Check sheet for the modelled part. Datum: model origin and axes. Units: mm. A direction names the side the tool comes from. Coordinates: 2 decimals unless noted, no trailing zeros. Write each loop counter-clockwise with the first axis right and the second up, starting at its lowest first coordinate (ties: lowest second). Pieces come first, ordered by that corner, then holes. Notation, with made-up numbers: (42, -30) - (79, -30) arc R5 ccw to (79, -23) - close; hole circle Ø3 at (15.25, 64). An arc over 180 degrees is marked (long way). Use one line per item in the form item = value. Start each with the question number.
1. Cross-section at A-A on y = -21. Record the boundary of the cut face in (x, z), then the cut area to 3 significant figures.
2. Go/stop test with flat-tipped pins: pin 1 Ø1 at (x, z) = (-9, 3.5) entering from +Y; pin 2 Ø5 at (x, y) = (7.5, -29) entering from -Z; pin 3 Ø2 at (x, z) = (14, 11) entering from +Y. Record where each tip stops, or that it passes through.
3. Cross-section at C-C on z = -7.5. Record the boundary of the cut face in (x, y).
4. Tool access check on faces 1 (the face through (17, -29, 5.625)), 2 (the face through (-4.5, -29, -18)), 3 (the face through (18.47, -27.986, 7.625)), 4 (the face through (5.36, -30.27, -1.29)). Record the directions out of +Z, -Z, +X, -X, +Y, -Y that give a thin tool (end or side, any length) a straight path to the whole face; none if there is none.
5. Cross-section at B-B on y = -11. Record the boundary of the cut face in (x, z).
6. Draft check along Z on faces 5 (the face through (6.31, -27.99, 5.84)), 6 (the face through (-8, -18.95, 2)), 7 (the face through (17, -29, 14.625)). Enter one of: +Z half, -Z half, draft (parallel to the pull), parting line (faces both ways), or undercut.
7. Scan lines: line 1 along Z through (x, y) = (7.5, -29.6); line 2 along X through (y, z) = (-30.95, -17.75); line 3 along Y through (x, z) = (11.5, -4.5). Record each from-to range of solid material in increasing order.
```python
from build123d import *

# Parameters (mm, degrees)
F0_R          = 1.5
F0_R_2        = 4.25
F1_DEPTH      = 3.5
F2_R          = 1.5
F2_W          = 9
F2_H          = 9
F2_R_2        = 1.6
F2_W_2        = 25
F2_H_2        = 3.5
F3_DEPTH      = 3.5
F3_DEPTH_BACK = 1
F4_R          = 1.6
F5_DEPTH      = 2
F6_R          = 2.9
F6_R_2        = 1.5
F7_DEPTH      = 2.5


# Not quite as in the source:
# - a feature names something its author has since deleted; it is built from what else it names


with BuildPart() as f1:
    # F0 (on Top) → F1 (new body)
    with BuildSketch(Plane.XY):
        with BuildLine():
            Line((-14.1, -30.5), (0, -30.5))
            Line((0, -30.5), (14.1, -30.5))
            Line((14.1, -30.5), (14.1, -12))
            Line((14.1, -12), (9.025382269, 3.044355416))
            ThreePointArc((9.025382269, 3.044355416), (0, 9.525), (-9.025382269, 3.044355416))
            Line((-9.025382269, 3.044355416), (-14.1, -12))
            Line((-14.1, -12), (-14.1, -30.5))
        make_face()
        Polygon((10.2, -27), (0, -27), (-10.2, -27), (-10.2, -18.95), (-5, -18.95), (-5, -9.525), (0, -9.525), (5, -9.525), (5, -18.95), (10.2, -18.95), align=None, mode=Mode.SUBTRACT)
        with Locations((-5.499261314, 3.175)):
            Circle(F0_R, mode=Mode.SUBTRACT)
        with Locations((0, -6.35)):
            Circle(F0_R, mode=Mode.SUBTRACT)
        Circle(F0_R_2, mode=Mode.SUBTRACT)
        with Locations((5.499261314, 3.175)):
            Circle(F0_R, mode=Mode.SUBTRACT)
    extrude(amount=F1_DEPTH)

    # F2 (on face) → F3 (join, two sides)
    with BuildSketch(Plane.XZ.offset(30.5)) as f3_sk:
        Polygon((12.5, 16.75), (-12.5, 16.75), (-12.5, 14.625), (-12.5, 5.625), (-12.5, 3.5), (12.5, 3.5), (12.5, 5.625), (12.5, 14.625), align=None)
        with Locations((-7.5, 6.75)):
            Circle(F2_R, mode=Mode.SUBTRACT)
        with Locations((7.5, 6.75)):
            Circle(F2_R, mode=Mode.SUBTRACT)
        Polygon((12.5, 0), (-12.5, 0), (-12.5, -13.25), (-4.5, -13.25), (4.5, -13.25), (12.5, -13.25), align=None)
        with Locations((-7.5, -3.25)):
            Circle(F2_R, mode=Mode.SUBTRACT)
        with Locations((7.5, -3.25)):
            Circle(F2_R, mode=Mode.SUBTRACT)
        with Locations((-17, 10.125)):
            Rectangle(F2_W, F2_H)
        with Locations((-17, 10.125)):
            Circle(F2_R_2, mode=Mode.SUBTRACT)
        with Locations((17, 10.125)):
            Rectangle(F2_W, F2_H)
        with Locations((17, 10.125)):
            Circle(F2_R_2, mode=Mode.SUBTRACT)
        with Locations((0, -17.75)):
            Rectangle(F2_W, F2_H)
        with Locations((0, -17.75)):
            Circle(F2_R_2, mode=Mode.SUBTRACT)
        with Locations((0, 1.75)):
            Rectangle(F2_W_2, F2_H_2)
    extrude(amount=-F3_DEPTH)
    extrude(f3_sk.sketch, amount=F3_DEPTH_BACK)

    # F4 (on face) → F5 (cut)
    with BuildSketch(Plane(origin=(0, -27, 0), x_dir=(-1, 0, 0), z_dir=(0, 1, 0))):
        Polygon((-19.9, 11.7993157806), (-19.9, 8.4506842194), (-17, 6.7763684387), (-14.1, 8.4506842194), (-14.1, 11.7993157806), (-17, 13.4736315613), align=None)
        with Locations((-17, 10.125)):
            Circle(F4_R, mode=Mode.SUBTRACT)
        Polygon((17, 13.4736315613), (14.1, 11.7993157806), (14.1, 8.4506842194), (17, 6.7763684387), (19.9, 8.4506842194), (19.9, 11.7993157806), align=None)
        with Locations((17, 10.125)):
            Circle(F4_R, mode=Mode.SUBTRACT)
        Polygon((1.6743157806, -14.85), (-1.6743157806, -14.85), (-3.3486315613, -17.75), (-1.6743157806, -20.65), (1.6743157806, -20.65), (3.3486315613, -17.75), align=None)
        with Locations((0, -17.75)):
            Circle(F4_R, mode=Mode.SUBTRACT)
    extrude(amount=-F5_DEPTH, mode=Mode.SUBTRACT)

    # F6 (on face) → F7 (cut)
    with BuildSketch(Plane.XZ.offset(31.5)):
        with Locations((-7.5, 6.75)):
            Circle(F6_R)
        with Locations((-7.5, 6.75)):
            Circle(F6_R_2, mode=Mode.SUBTRACT)
        with Locations((7.5, 6.75)):
            Circle(F6_R)
        with Locations((7.5, 6.75)):
            Circle(F6_R_2, mode=Mode.SUBTRACT)
        with Locations((7.5, -3.25)):
            Circle(F6_R)
        with Locations((7.5, -3.25)):
            Circle(F6_R_2, mode=Mode.SUBTRACT)
        with Locations((-7.5, -3.25)):
            Circle(F6_R)
        with Locations((-7.5, -3.25)):
            Circle(F6_R_2, mode=Mode.SUBTRACT)
    extrude(amount=-F7_DEPTH, mode=Mode.SUBTRACT)


solid = f1.part
```
Final values:
q1.outline = (-14.1, 0) - (-10.2, 0) - (-10.2, 3.5) - (-14.1, 3.5) - close; (10.2, 0) - (14.1, 0) - (14.1, 3.5) - (10.2, 3.5) - close
q1.area = 27.3 mm²
q2.pin_1 = 4.3
q2.pin_2 = -13.25
q2.pin_3 = -27
q3.outline = (-12.5, -31.5) - (12.5, -31.5) - (12.5, -27) - (-12.5, -27) - close
q4.face_1 = +X, +Y, -Y
q4.face_2 = -Z, -X, +Y, -Y
q4.face_3 = +Y
q4.face_4 = -Y
q5.outline = (-13.76, 0) - (-5, 0) - (-5, 3.5) - (-13.76, 3.5) - close; (5, 0) - (13.76, 0) - (13.76, 3.5) - (5, 3.5) - close
q6.face_5 = undercut
q6.face_6 = draft
q6.face_7 = +Z half
q7.line_1 = -13.25 to -6.15, -0.35 to 3.85, 9.65 to 16.75
q7.line_2 = -4.5 to -1.6, 1.6 to 4.5
q7.line_3 = -31.5 to -27
